```python
from build123d import *

# Parameters (mm, degrees)
SKETCH_1_R          = 5
EXTRUDE_1_DEPTH     = 18
SKETCH_3_R          = 3.1
CUT_EXTRUDE_1_DEPTH = 17
EXTRUDE_2_DEPTH     = 12
SKETCH_8_R          = 3.9
EXTRUDE_4_DEPTH     = 5
SKETCH_9_R          = 2.6
CUT_EXTRUDE_2_DEPTH = 5
EXTRUDE_5_DEPTH     = 3
FILLET_1_R          = 0.2
CHAMFER_1_SIZE      = 0.5


with BuildPart() as part:
    # 草图1 → 凸台-拉伸1 (new body)
    with BuildSketch(Plane(origin=(0, 0, 0), x_dir=(0, 0, -1), z_dir=(1, 0, 0))):
        Circle(SKETCH_1_R)
    extrude(amount=EXTRUDE_1_DEPTH)

    # 草图3 → 切除-拉伸1 (cut)
    with BuildSketch(Plane(origin=(18, 0, 0), x_dir=(0, 0, -1), z_dir=(1, 0, 0))):
        Circle(SKETCH_3_R)
    extrude(amount=-CUT_EXTRUDE_1_DEPTH, mode=Mode.SUBTRACT)

    # 草图5 → 凸台-拉伸2 (add)
    with BuildSketch(Plane(origin=(1, 0, 0), x_dir=(0, 0, -1), z_dir=(1, 0, 0))):
        with BuildLine():
            Line((-1.688194302, 2.6), (1.688194302, 2.6))
            Line((1.688194302, 2.6), (1.688194302, 5.234500931))
            ThreePointArc((1.688194302, 5.234500931), (0, 5.5), (-1.688194302, 5.234500931))
            Line((-1.688194302, 5.234500931), (-1.688194302, 2.6))
        make_face()
    extrude(amount=EXTRUDE_2_DEPTH)

    # 草图8 → 凸台-拉伸4 (add)
    with BuildSketch(Plane.ZY):
        Circle(SKETCH_8_R)
    extrude(amount=EXTRUDE_4_DEPTH)

    # 草图9 → 切除-拉伸2 (cut)
    with BuildSketch(Plane.ZY.offset(5)):
        Circle(SKETCH_9_R)
    extrude(amount=-CUT_EXTRUDE_2_DEPTH, mode=Mode.SUBTRACT)

    # 草图10 → 凸台-拉伸5 (add)
    with BuildSketch(Plane.ZY):
        Polygon((0.66395281, 1.15), (-0.66395281, 1.15), (-1.327905619, 0), (-0.66395281, -1.15), (0.66395281, -1.15), (1.327905619, 0), align=None)
    extrude(amount=EXTRUDE_5_DEPTH)

    # 圆角1
    fillet_1_edges = [part.edges().sort_by_distance(p)[0] for p in [
        (7, 4.70637865, 1.688194302),
        (7, 5.234500931, 1.688194302),
        (7, 4.70637865, -1.688194302),
        (7, 5.234500931, -1.688194302),
    ]]
    fillet(fillet_1_edges, radius=FILLET_1_R)

    # 倒角1
    # the kernel refuses this chamfer: 0.5 mm, written as the material it takes off along each edge
    with BuildSketch(Plane(origin=(13, 0, 0), x_dir=(0, 0.8686030413593419, -0.4955085837211114), z_dir=(0, -0.4955085837211114, -0.8686030413593419))) as chamfer_1_piece_1:
        Polygon((5.5, -CHAMFER_1_SIZE), (5.5 - CHAMFER_1_SIZE, 0), (5.5, 0), align=None)
    revolve(axis=Axis((13, 0, 0), (1, 0, 0)), revolution_arc=59.40658503, mode=Mode.SUBTRACT)
    with BuildSketch(Plane(origin=(1, 0, 0), x_dir=(0, 0.8686030413593416, -0.4955085837211117), z_dir=(0, -0.4955085837211117, -0.8686030413593416))) as chamfer_1_piece_2:
        Polygon((5.5 - CHAMFER_1_SIZE, 0), (5.5, CHAMFER_1_SIZE), (5.5, 0), align=None)
    revolve(axis=Axis((1, 0, 0), (1, 0, 0)), revolution_arc=59.40658503, mode=Mode.SUBTRACT)
    with BuildSketch(Plane(origin=(13, 2.6, 2.974035796), x_dir=(0.027495876610585623, 0.9996219169112968, 0), z_dir=(0, 0, -1))) as chamfer_1_piece_3_section:
        Polygon((CHAMFER_1_SIZE * 0.999621916911, -CHAMFER_1_SIZE * 0.0274958766106), (-CHAMFER_1_SIZE * 0.0274958766106, -CHAMFER_1_SIZE * 0.999621916911), (0, 0), align=None)
    chamfer_1_piece_3 = extrude(amount=5.948071591, mode=Mode.PRIVATE)
    chamfer_1_piece_3 = chamfer_1_piece_3 & Plane(origin=(12.821912141, 0, 0), x_dir=(0, 0, -1), z_dir=(1, 0, 0)) * Cylinder(3.1, 14, mode=Mode.PRIVATE)
    add(chamfer_1_piece_3, mode=Mode.SUBTRACT)


solid = part.part
```
For this review, take the finished solid that the model builds, in its own axes (mm). A direction names the side the tool comes from. Round coordinates to 2 decimals unless told otherwise and drop trailing zeros. Write each loop counter-clockwise with the first axis right and the second up, starting at its lowest first coordinate (ties: lowest second). Pieces come first, ordered by that corner, then holes. Notation, with made-up numbers: (64.25, -21.5) - (72.25, -21.5) arc R16 cw to (72.25, -11.5) - close; hole circle Ø9 at (-29, 79.5). An arc over 180 degrees is marked (long way). Use CSV: the item, a comma, the result in double quotes.
1) Add section C-C on z = 0. Write out the cut boundary in (x, y), and give its area (3 significant figures).
Conclusion:
outline,"(-5, -3.9) - (0, -3.9) - (0, -5) - (18, -5) - (18, -3.1) - (1, -3.1) - (1, 2.6) - (12.5, 2.6) - (13, 3.1) - (18, 3.1) - (18, 5) - (13, 5) - (12.5, 5.5) - (1.5, 5.5) - (1, 5) - (0, 5) - (0, 3.9) - (-5, 3.9) - (-5, 2.6) - (0, 2.6) - (0, 1.15) - (-3, 1.15) - (-3, -1.15) - (0, -1.15) - (0, -2.6) - (-5, -2.6) - close"
area,"106 mm^2"
2) Wall thickness on line 1 along Y through (x, z) = (-1.7, 0); line 2 along X through (y, z) = (1.5, -2.5); line 3 along Y through (x, z) = (6, 0): over which ranges is each line inside the solid? List them lowest first. Write a range as from..to.
Conclusion:
line 1,"y = -3.9..-2.6, -1.15..1.15, 2.6..3.9"
line 2,"x = -5..1"
line 3,"y = -5..-3.1, 2.6..5.5"
3) The part is to be moulded in two halves that separate along Y. For faces 1 (the flat face through (-1.48, -0.57, -1)), 2 (the cylindrical face through (-2.46, 2.64, -2.87)), 3 (the conical face through (1.2, 5.2, 0)), say which applies: pulls with the +Y half, pulls with the -Y half, needs draft (parallel to the pull), parting line crosses it, or undercut.
Conclusion:
face 1,"undercut"
face 2,"parting line crosses it"
face 3,"pulls with the +Y half"
4) Add section D-D on y = -0.75. Write out the cut boundary in (x, z), and give its area (3 significant figures).
Conclusion:
outline,"(-5, -3.83) - (0, -3.83) - (0, -4.94) - (18, -4.94) - (18, -3.01) - (1, -3.01) - (1, 3.01) - (18, 3.01) - (18, 4.94) - (0, 4.94) - (0, 3.83) - (-5, 3.83) - (-5, 2.49) - (0, 2.49) - (0, 0.89) - (-3, 0.89) - (-3, -0.89) - (0, -0.89) - (0, -2.49) - (-5, -2.49) - close"
area,"94.4 mm^2"
5) Add section A-A on x = -2. Write out the cut boundary in (y, z), and give its area (3 significant figures).
Conclusion:
outline,"circle Ø7.8 at (0, 0); (-1.15, -0.66) - (0, -1.33) - (1.15, -0.66) - (1.15, 0.66) - (0, 1.33) - (-1.15, 0.66) - close; hole circle Ø5.2 at (0, 0)"
area,"31.1 mm^2"
6) Clearance check with flat-ended pins moving along their axes: pin 1 Ø1 at (y, z) = (0, 1.5) entering from -X; pin 2 Ø3 at (x, y) = (2.5, -2) entering from +Z; pin 3 Ø0.7 at (x, z) = (-1.5, 0) entering from -Y. State where each tip first meets the part, or that it passes through.
Conclusion:
pin 1,"stops at x = -3"
pin 2,"stops at z = 4.97"
pin 3,"stops at y = -3.9"
7) Add section B-B on x = 3. Write out the cut boundary in (y, z).
Conclusion:
outline,"(4.66, -1.82) arc R0.2 cw to (4.85, -1.69) - (5.09, -1.69) arc R0.2 ccw to (5.28, -1.54) arc R5.5 ccw to (5.28, 1.54) arc R0.2 ccw to (5.09, 1.69) - (4.85, 1.69) arc R0.2 cw to (4.66, 1.82) arc R5 ccw (long way) to start; hole (2.6, -1.69) - (2.6, 1.69) arc R3.1 ccw (long way) to start"
8) For faces 4 (the flat face through (-1, 1.15, 0)), 5 (the cylindrical face through (6.9, 5.5, 0)), 6 (the flat face through (1, 0, 0)), list the 3-axis set-ups (+Z, -Z, +X, -X, +Y, -Y) from which the entire face can be reached by the end or side of a thin tool; tool diameter is ignored.
Conclusion:
face 4,"-X"
face 5,"+X, -X, +Y"
face 6,"+X"
